```python
from build123d import *

# Parameters (mm, degrees)
SKETCH1_R           = 2.5
BOSS_EXTRUDE1_DEPTH = 50
SCALE_2_SCALE       = 3
SCALE_3_SCALE       = 6
SCALE_5_SCALE       = 2
SCALE_6_SCALE       = 0.25
SCALE_7_SCALE       = 0.125
SCALE_8_SCALE       = 0.25
SCALE_9_SCALE       = 4
SCALE_10_SCALE      = 4
OTHER_START         = -17.55
OTHER_1_OUTLINE_R   = 5
OTHER_1_DEPTH       = 10
SCALE_11_SCALE      = 0.111111111


# Read off the part's stored shape, not the designer's step: 孔1
with BuildPart() as part:
    # Sketch1 → Boss-Extrude1 (new body)
    with BuildSketch(Plane.XY):
        with BuildLine():
            Line((2.839339828, 3.9), (5.5, 6.560660172))
            Line((5.5, 6.560660172), (5.5, 8.2))
            Line((5.5, 8.2), (3.1, 8.2))
            Line((3.1, 8.2), (3.1, 9.5))
            Line((3.1, 9.5), (3.6, 9.5))
            Line((3.6, 9.5), (3.6, 10))
            Line((3.6, 10), (8.5, 10))
            ThreePointArc((8.5, 10), (9.560660172, 9.560660172), (10, 8.5))
            Line((10, 8.5), (10, 3.6))
            Line((10, 3.6), (9.5, 3.6))
            Line((9.5, 3.6), (9.5, 3.1))
            Line((9.5, 3.1), (8.2, 3.1))
            Line((8.2, 3.1), (8.2, 5.5))
            Line((8.2, 5.5), (6.560660172, 5.5))
            Line((6.560660172, 5.5), (3.9, 2.839339828))
            Line((3.9, 2.839339828), (3.9, -2.839339828))
            Line((3.9, -2.839339828), (6.560660172, -5.5))
            Line((6.560660172, -5.5), (8.2, -5.5))
            Line((8.2, -5.5), (8.2, -3.1))
            Line((8.2, -3.1), (9.5, -3.1))
            Line((9.5, -3.1), (9.5, -3.6))
            Line((9.5, -3.6), (10, -3.6))
            Line((10, -3.6), (10, -8.5))
            ThreePointArc((10, -8.5), (9.560660172, -9.560660172), (8.5, -10))
            Line((8.5, -10), (3.6, -10))
            Line((3.6, -10), (3.6, -9.5))
            Line((3.6, -9.5), (3.1, -9.5))
            Line((3.1, -9.5), (3.1, -8.2))
            Line((3.1, -8.2), (5.5, -8.2))
            Line((5.5, -8.2), (5.5, -6.560660172))
            Line((5.5, -6.560660172), (2.839339828, -3.9))
            Line((2.839339828, -3.9), (-2.839339828, -3.9))
            Line((-2.839339828, -3.9), (-5.5, -6.560660172))
            Line((-5.5, -6.560660172), (-5.5, -8.2))
            Line((-5.5, -8.2), (-3.1, -8.2))
            Line((-3.1, -8.2), (-3.1, -9.5))
            Line((-3.1, -9.5), (-3.6, -9.5))
            Line((-3.6, -9.5), (-3.6, -10))
            Line((-3.6, -10), (-8.5, -10))
            ThreePointArc((-8.5, -10), (-9.560660172, -9.560660172), (-10, -8.5))
            Line((-10, -8.5), (-10, -3.6))
            Line((-10, -3.6), (-9.5, -3.6))
            Line((-9.5, -3.6), (-9.5, -3.1))
            Line((-9.5, -3.1), (-8.2, -3.1))
            Line((-8.2, -3.1), (-8.2, -5.5))
            Line((-8.2, -5.5), (-6.560660172, -5.5))
            Line((-6.560660172, -5.5), (-3.9, -2.839339828))
            Line((-3.9, -2.839339828), (-3.9, 2.839339828))
            Line((-3.9, 2.839339828), (-6.560660172, 5.5))
            Line((-6.560660172, 5.5), (-8.2, 5.5))
            Line((-8.2, 5.5), (-8.2, 3.1))
            Line((-8.2, 3.1), (-9.5, 3.1))
            Line((-9.5, 3.1), (-9.5, 3.6))
            Line((-9.5, 3.6), (-10, 3.6))
            Line((-10, 3.6), (-10, 8.5))
            ThreePointArc((-10, 8.5), (-9.560660172, 9.560660172), (-8.5, 10))
            Line((-8.5, 10), (-3.6, 10))
            Line((-3.6, 10), (-3.6, 9.5))
            Line((-3.6, 9.5), (-3.1, 9.5))
            Line((-3.1, 9.5), (-3.1, 8.2))
            Line((-3.1, 8.2), (-5.5, 8.2))
            Line((-5.5, 8.2), (-5.5, 6.560660172))
            Line((-5.5, 6.560660172), (-2.839339828, 3.9))
            Line((-2.839339828, 3.9), (2.839339828, 3.9))
        make_face()
        with Locations((0, 0.235847297)):
            Circle(SKETCH1_R, mode=Mode.SUBTRACT)
    extrude(amount=BOSS_EXTRUDE1_DEPTH)


with BuildPart() as part_1:
    # 缩放比例2: scaled about (0, -0.027095247, 25)
    add(part.part.scale(SCALE_2_SCALE).moved(Location((0, 0.054190494, -50))))


with BuildPart() as part_2:
    # 缩放比例3: scaled about (0, -0.027095247, 25)
    add(part_1.part.scale(SCALE_3_SCALE).moved(Location((0, 0.135476235, -125))))


with BuildPart() as part_3:
    # 缩放比例5: scaled about (0, -0.027095249, 25)
    add(part_2.part.scale(SCALE_5_SCALE).moved(Location((0, 0.027095249, -25))))


with BuildPart() as part_4:
    # 缩放比例6: scaled about (0, -0.027095249, 25)
    add(part_3.part.scale(SCALE_6_SCALE).moved(Location((0, -0.020321437, 18.75))))


with BuildPart() as part_5:
    # 缩放比例7: scaled about (0, -0.027095249, 25)
    add(part_4.part.scale(SCALE_7_SCALE).moved(Location((0, -0.023708343, 21.875))))


with BuildPart() as part_6:
    # 缩放比例8: scaled about (0, -0.027095249, 25)
    add(part_5.part.scale(SCALE_8_SCALE).moved(Location((0, -0.020321437, 18.75))))


with BuildPart() as part_7:
    # 缩放比例9: scaled about (0, -0.027095249, 25)
    add(part_6.part.scale(SCALE_9_SCALE).moved(Location((0, 0.081285747, -75))))


with BuildPart() as part_8:
    # 缩放比例10: scaled about (0, -0.027095249, 25)
    add(part_7.part.scale(SCALE_10_SCALE).moved(Location((0, 0.081285747, -75))))

    # 孔1 outline → 孔1 (cut)
    with BuildSketch(Plane.YZ.offset(OTHER_START)):
        with Locations((7.344833538, 1.297306883)):
            Circle(OTHER_1_OUTLINE_R)
    extrude(amount=OTHER_1_DEPTH, mode=Mode.SUBTRACT)


with BuildPart() as part_9:
    # 缩放比例11: scaled about (0.011151362, -0.033595737, 25.019879338)
    add(part_8.part.scale(SCALE_11_SCALE).moved(Location((0.009912322, -0.029862877, 22.239892745))))


solid = part_9.part
```
Input: part model. Units: mm. Frame: model coordinates. A direction names the side the tool comes from. Round coordinates to 2 decimals unless told otherwise and drop trailing zeros. Loops run counter-clockwise (first coordinate to the right, second up) from the corner with the lowest first, then second, coordinate; pieces in that order, holes last. Notation, with made-up numbers: M 11.25,57 L 25.25,57 A12 ccw 25.25,76 Z; hole C -35,6.5 d11. An arc over 180 degrees is marked long. Answer in a Markdown table with one row per item. Add a question column.
1. Section A-A (x = -3). Output: boundary loops of the cut face in (y, z).
2. Section D-D (y = 2.25). Output: boundary loops of the cut face in (x, z).
3. Section C-C (x = 2.5). Output: boundary loops of the cut face in (y, z), and give its area (3 significant figures).
4. Section B-B (y = -0.5). Output: boundary loops of the cut face in (x, z), and give its area (3 significant figures).
5. Contact query for flat-ended pins moving along their axis: pin 1 (2 mm diameter, centred on x = 0.01, y = 0.1, fed in from +Z); pin 2 (0.7 mm diameter, centred on y = 0.79, z = 22.38, fed in from +X). Output: stop coordinate, or through.
6. Ray query, probe 1 along X at (y, z) = (-3.5, 28.75); probe 2 along Y at (x, z) = (-3.75, 14.25); probe 3 along X at (y, z) = (1.75, 24.75). Return the intervals inside material, ascending.
7. Set-up query: faces 5 (the face through (5.01, 3, 25)), 6 (the face through (3.7, 2.731, 24.8)), 7 (the face through (0, 1.931, 25)). Return all of +Z, -Z, +X, -X, +Y, -Y with unobstructed straight access to the full face (end or side cutting, diameter ignored); none if empty.
8. Mould query, pull axis Y, two halves, no side actions, for faces 1 (the face through (-2.6, 2.06, 24.84)), 2 (the face through (2.1, 2.6, 24.8)), 3 (the face through (-3, -5.019, 25)), 4 (the face through (1.2, 1.2, 12.518)). Classes: released by +Y, released by -Y, zero draft, split by the parting line, or undercut.
Values follow:
| question | item | result |
|---|---|---|
| 1 | outline | M -5.02,12.52 L -2.5,12.52 L -2.5,37.52 L -5.02,37.52 Z; M 2.46,12.52 L 4.98,12.52 L 4.98,37.52 L 2.46,37.52 Z |
| 2 | outline | M -4.99,12.52 L -4.09,12.52 L -4.09,37.52 L -4.99,37.52 Z; M -2.79,12.52 L -1.73,12.52 L -1.73,37.52 L -2.79,37.52 Z; M 1.75,12.52 L 2.81,12.52 L 2.81,37.52 L 1.75,37.52 Z; M 4.11,12.52 L 5.01,12.52 L 5.01,37.52 L 4.11,37.52 Z |
| 3 | outline | M -5.02,12.52 L -4.12,12.52 L -4.12,37.52 L -5.02,37.52 Z; M -3.04,12.52 L -1.98,12.52 L -1.98,37.52 L -3.04,37.52 Z; M 1.94,12.52 L 3,12.52 L 3,37.52 L 1.94,37.52 Z; M 4.08,12.52 L 4.98,12.52 L 4.98,37.52 L 4.08,37.52 Z |
| 3 | area | 98.0 mm^2 |
| 4 | outline | M -1.94,12.52 L -1.09,12.52 L -1.09,37.52 L -1.94,37.52 Z; M 1.11,12.52 L 1.96,12.52 L 1.96,37.52 L 1.11,37.52 Z |
| 4 | area | 42.6 mm^2 |
| 5 | pin 1 | through |
| 5 | pin 2 | x = 1.96 |
| 6 | probe 1 | -4.99 to -2.74, 2.76 to 5.01 |
| 6 | probe 2 | -5.02 to -2.77, 2.73 to 4.98 |
| 6 | probe 3 | -4.74 to -4.09, -2.29 to 2.31, 4.11 to 4.76 |
| 7 | face 5 | +Z, -Z, +X, +Y, -Y |
| 7 | face 6 | +Z, -Z |
| 7 | face 7 | +Z, -Z, +Y |
| 8 | face 1 | undercut |
| 8 | face 2 | undercut |
| 8 | face 3 | released by -Y |
| 8 | face 4 | zero draft |
